Check sheet for the drawn part. Datum: minimum x, y, z corner. Units: mm. Coordinates: 2 decimals unless noted, no trailing zeros. Order: outer loops, then holes, each group sorted by start corner. A loop starts at its lowest first (then second) coordinate and runs counter-clockwise, first axis right, second up. Notation, with made-up numbers: (-28, -38) -> (-11, -38) arc R23 cw to (-11, -21) -> close; hole circle Ø10 at (39, 41). An arc over 180 degrees is marked (long way). Write item = value, one per line. Start each with the question number.
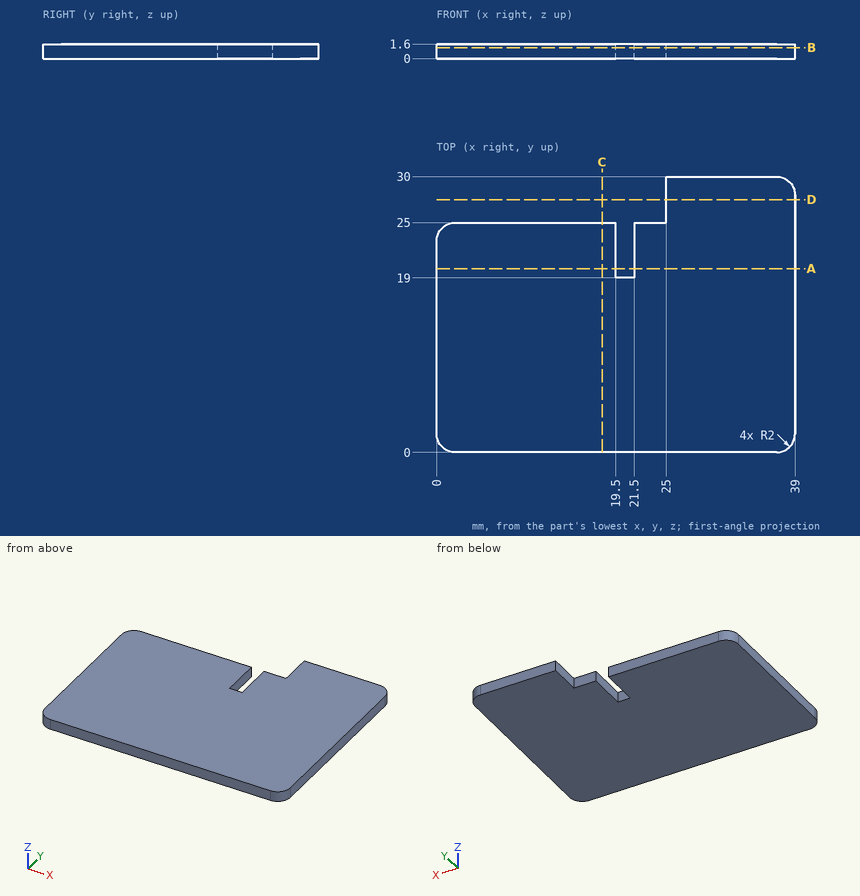
Item 1: Thickness scan on line 1 (X direction, y = 22.5, z = 0.8); line 2 (Y direction, x = 2, z = 0.15); line 3 (X direction, y = 23.5, z = 0.7). Record the ranges inside material, lowest first.
Item 2: Section check C-C (x = 18). Record the boundary of the cut face in (y, z), then the cut area to 3 significant figures.
Item 3: Section check D-D (y = 27.5). Record the boundary of the cut face in (x, z).
Item 4: Section check A-A (y = 20). Record the boundary of the cut face in (x, z), then the cut area to 3 significant figures.
Item 5: Section check B-B (z = 1.2). Record the boundary of the cut face in (x, y), then the cut area to 3 significant figures.
Item 6: Gauge pin test, flat ends, axial feed: P1, Ø0.8, axis at x = 22.5, z = 0.5, coming from the +Y side; P2, Ø0.5, axis at y = 27, z = 1, coming from the -X side. Record the tip position at first contact, or that the pin passes through.
Filled sheet:
q1.line_1 = 0 to 19.5, 21.5 to 39
q1.line_2 = 0 to 25
q1.line_3 = 0.06 to 19.5, 21.5 to 39
q2.outline = (0, 0) -> (25, 0) -> (25, 1.6) -> (0, 1.6) -> close
q2.area = 40.0 mm^2
q3.outline = (25, 0) -> (39, 0) -> (39, 1.6) -> (25, 1.6) -> close
q4.outline = (0, 0) -> (19.5, 0) -> (19.5, 1.6) -> (0, 1.6) -> close; (21.5, 0) -> (39, 0) -> (39, 1.6) -> (21.5, 1.6) -> close
q4.area = 59.2 mm^2
q5.outline = (0, 2) arc R2 ccw to (2, 0) -> (37, 0) arc R2 ccw to (39, 2) -> (39, 28) arc R2 ccw to (37, 30) -> (25, 30) -> (25, 25) -> (21.5, 25) -> (21.5, 19) -> (19.5, 19) -> (19.5, 25) -> (2, 25) arc R2 ccw to (0, 23) -> close
q5.area = 1,030 mm^2
q6.P1 = 25
q6.P2 = 25
